Here's how the part is built. I have some questions about the finished solid (model axes, mm). Face numbers are marked on the shaded views. A direction names the side the tool comes from. Round coordinates to 2 decimals unless told otherwise and drop trailing zeros. Order: outer loops, then holes, each group sorted by start corner. A loop starts at its lowest first (then second) coordinate and runs counter-clockwise, first axis right, second up. Notation, with made-up numbers: (16.25, 33.5) -> (63.25, 33.5) arc R19 cw to (63.25, 65.5) -> close; hole circle Ø6 at (37, 14.25). An arc over 180 degrees is marked (long way). Answer in a Markdown table with one row per item.
```python
from build123d import *

# Parameters (mm, degrees)
F0_W     = 12.0142
F0_H     = 5.7658
F1_DEPTH = 5.08
F2_W     = 14.5542
F2_H     = 8.509
F3_DEPTH = 1.27
F4_R     = 0.762


with BuildPart() as f1:
    # F0 (on Top) → F1 (new body)
    with BuildSketch(Plane.XY):
        Rectangle(F0_W, F0_H)
    extrude(amount=F1_DEPTH)

    # F2 (on Top) → F3 (join)
    with BuildSketch(Plane.XY):
        Rectangle(F2_W, F2_H)
    extrude(amount=-F3_DEPTH)

    # F4
    f4_edges = [f1.edges().sort_by_distance(p)[0] for p in [
        (6.0071, 0, 5.08),
        (0, 2.8829, 5.08),
        (-6.0071, 0, 5.08),
        (0, -2.8829, 5.08),
    ]]
    fillet(f4_edges, radius=F4_R)


solid = f1.part
```
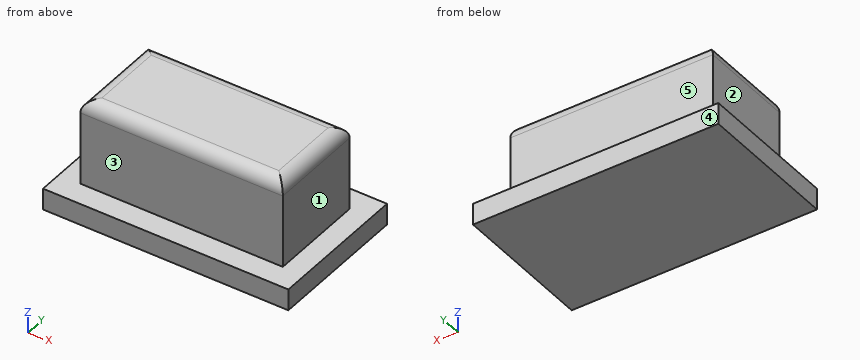
1. Suppose I cut it at B-B on y = 0. Write out the boundary of the cut face in (x, z), then the cut area to 3 significant figures.
Numbers:
| item | result |
|---|---|
| outline | (-7.28, -1.27) -> (7.28, -1.27) -> (7.28, 0) -> (6.01, 0) -> (6.01, 4.32) arc R0.76 ccw to (5.25, 5.08) -> (-5.25, 5.08) arc R0.76 ccw to (-6.01, 4.32) -> (-6.01, 0) -> (-7.28, 0) -> close |
| area | 79.3 mm2 |
2. Suppose I cut it at A-A on x = -2.5. Write out the boundary of the cut face in (y, z), then the cut area to 3 significant figures.
Numbers:
| item | result |
|---|---|
| outline | (-4.25, -1.27) -> (4.25, -1.27) -> (4.25, 0) -> (2.88, 0) -> (2.88, 4.32) arc R0.76 ccw to (2.12, 5.08) -> (-2.12, 5.08) arc R0.76 ccw to (-2.88, 4.32) -> (-2.88, 0) -> (-4.25, 0) -> close |
| area | 39.8 mm2 |
3. For the marked faces 1, 2, 3, 4 and 5, which set-ups out of +Z, -Z, +X, -X, +Y, -Y let a thin tool reach every point of the face, with its end or its side?
Numbers:
| item | result |
|---|---|
| face 1 | +Z, +X, +Y, -Y |
| face 2 | +Z, -X, +Y, -Y |
| face 3 | +Z, +X, -X, -Y |
| face 4 | +Z, -Z, +X, -X, +Y |
| face 5 | +Z, +X, -X, +Y |
4. Suppose I cut it at D-D on y = 3.25. Write out the boundary of the cut face in (x, z), then the cut area to 3 significant figures.
Numbers:
| item | result |
|---|---|
| outline | (-7.28, -1.27) -> (7.28, -1.27) -> (7.28, 0) -> (-7.28, 0) -> close |
| area | 18.5 mm2 |
5. Suppose I cut it at C-C on z = 0.75. Write out the boundary of the cut face in (x, y), then the cut area to 3 significant figures.
Numbers:
| item | result |
|---|---|
| outline | (-6.01, -2.88) -> (6.01, -2.88) -> (6.01, 2.88) -> (-6.01, 2.88) -> close |
| area | 69.3 mm2 |
6. For pin 1 Ø1.5 at (y, z) = (-3.5, 3) entering from -X; pin 2 Ø3.5 at (x, z) = (-1, 1.5) entering from +Y; pin 3 Ø2 at (y, z) = (-1.5, 2) entering from +X; pin 4 Ø1 at (x, z) = (-2, 4) entering from +Y, each with a flat end and sliding along its axis, tell me the tip position at first contact or that it passes through.
Numbers:
| item | result |
|---|---|
| pin 1 | stops at x = -6.01 |
| pin 2 | stops at y = 4.25 |
| pin 3 | stops at x = 6.01 |
| pin 4 | stops at y = 2.88 |
7. Please list where these lines run through material, in increasing order: line 1 along X through (y, z) = (-0.5, 1.75); line 2 along Z through (x, y) = (5.25, 3.5); line 3 along Y through (x, z) = (0, 0.75).
Numbers:
| item | result |
|---|---|
| line 1 | x = -6.01 to 6.01 |
| line 2 | z = -1.27 to 0 |
| line 3 | y = -2.88 to 2.88 |
